Geometry: final body of the model. Coordinates: model frame, mm. Face numbers are marked on the shaded views. A direction names the side the tool comes from. Give positions to 0.01 mm unless a question says otherwise; leave off trailing zeros. Write each loop counter-clockwise with the first axis right and the second up, starting at its lowest first coordinate (ties: lowest second). Pieces come first, ordered by that corner, then holes.
Autodesk Inventor part; units mm, degrees
ref_plane "YZ Plane" through (0, 0, 0) normal (1, 0, 0) x (0, 1, 0)
ref_plane "XZ Plane" through (0, 0, 0) normal (0, 1, 0) x (-1, 0, 0)
ref_plane "XY Plane" through (0, 0, 0) normal (0, 0, 1) x (1, 0, 0)
sketch "Sketch1" plane through (0, 0, 0) normal (0, 0, 1) x (1, 0, 0)
  line L0 (0, 0) -> (0, 40)
  dimension "d0" = 40
sketch "Sketch2" plane through (0, 0, 0) normal (0, 1, 0) x (-1, 0, 0)
  circle A0 centre (0, 0) radius 15
  dimension "d3" = 30
sweep "Sweep1" add profiles "Sketch2" path "Sketch1"
sketch "Sketch4" plane through (0, 0, 0) normal (1, 0, 0) x (0, 1, 0)
  line L0 (0, 17.5) -> (0, -17.5) construction
  line L1 (10, 17.5) -> (10, -17.5)
  line L2 (-10, -17.5) -> (-10, 17.5)
  arc A0 (10, 17.5) -> (-10, 17.5) centre (0, 17.5) ccw
  arc A1 (-10, -17.5) -> (10, -17.5) centre (0, -17.5) ccw
  line L3 (-10, 0) -> (10, 0)
  point P0 (0, 0)
  dimension "d9" = 35
  dimension "d10" = 10
revolve "Revolution1" add sketch "Sketch4" angle 360 about axis through (0, -10, 0) along (0, 1, 0) contours L1 L3 L2 A0
sketch "Sketch5" plane through (0, 0, 0) normal (0, 0, 1) x (1, 0, 0)
  line L0 (-30, 40) -> (30, 40)
  line L1 (30, 40) -> (30, 120)
  line L2 (30, 120) -> (-30, 120)
  line L3 (-30, 120) -> (-30, 40)
  circle A0 centre (0, 90) radius 12.5
  line L4 (0, 0) -> (0, 40) construction
  line L5 (0, 90) -> (0, 40)
  dimension "d12" = 90
  dimension "d13" = 25
  dimension "d14" = 60
  dimension "d15" = 30
extrude "Extrusion1" add sketch "Sketch5" along normal mid plane 80
sketch "Sketch7" plane through (-30, 40, 40) normal (-1, 0, 0) x (0, 0, 1)
  line L0 (-80, 80) -> (0, 80) construction
  line L1 (-65, 80) -> (-15, 80)
  line L2 (-15, 80) -> (-15, 20)
  line L3 (-15, 20) -> (-65, 20)
  line L4 (-65, 20) -> (-65, 80)
  line L5 (-80, 37.5) -> (-80, 62.5) construction
  line L6 (0, 62.5) -> (0, 37.5) construction
  line L7 (-80, 0) -> (-80, 80) construction
  line L8 (-80, 50) -> (0, 50) construction
  line L9 (0, 80) -> (0, 0) construction
  line L10 (-40, 50) -> (-40, 0) construction
  point P0 (-40, -40)
  dimension "d18" = 30
  dimension "d19" = 50
  dimension "d20" = 25
  dimension "d21" = 90
fillet "Fillet1" radius 10 13 edges at (-30, 80, 40) (30, 80, 40) (-30, 80, -40) (30, 80, -40) (-30, 40, 0) (0, 40, -40) (0, 40, 40) (30, 40, 0) (15, 40, 0) (-30, 120, 0) (0, 120, 40) (30, 120, 0) (0, 120, -40)
extrude "Extrusion2" cut sketch "Sketch7" against normal through all
equation "\"d20\" = 0.5 * d19"
properties part number "Elo-Bola Longo"
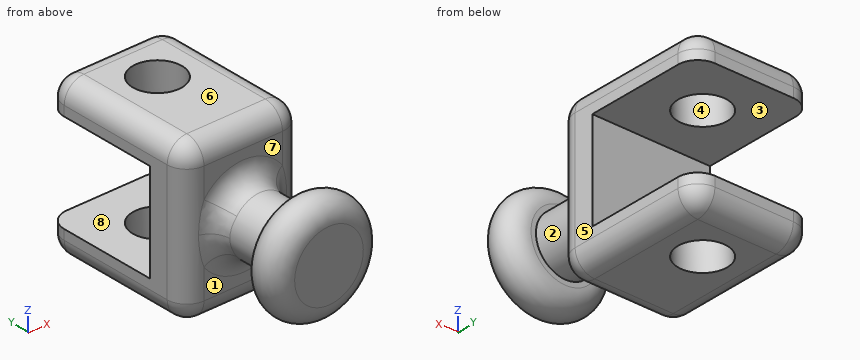
Q1. Ray query, line 1 along Z through (x, y) = (-13, 87); line 2 along Y through (x, z) = (0, 29); line 3 along X through (y, z) = (90, 28). Return the intervals inside material, ascending.
Filled sheet:
line 1: z = -40 to -25, 25 to 40
line 2: y = 40 to 77.5, 102.5 to 120
line 3: x = -30 to -12.5, 12.5 to 30
Q2. Section D-D on y = 25. Output: boundary loops of the cut face in (x, z).
Filled sheet:
outline: circle Ø30 at (0, 0)
Q3. Access query for the marked faces 1, 2, 3, 4 and 5. Directions: +Z, -Z, +X, -X, +Y, -Y. A direction counts if a zero-diameter tool reaches every point of the face in a straight line with its end or side. Return the directions, or none.
Filled sheet:
face 1: -Z
face 2: none
face 3: +X, -X, +Y
face 4: +Z, -Z
face 5: +Z, -Z, +X, +Y, -Y
Q4. Section B-B on x = 0. Count the separate pieces of the cut face and the enclosed holes in it, plus the area to 3 significant figures.
Filled sheet:
separate pieces: 3
enclosed holes: 0
area: 4,520 mm2
Q5. Section C-C on z = 32.5. Output: boundary loops of the cut face in (x, y), plus the area to 3 significant figures.
Filled sheet:
outline: (-29.68, 50) arc R9.68 ccw to (-20, 40.32) - (20, 40.32) arc R9.68 ccw to (29.68, 50) - (29.68, 110) arc R9.68 ccw to (20, 119.68) - (-20, 119.68) arc R9.68 ccw to (-29.68, 110) - close; hole circle Ø25 at (0, 90)
area: 4,140 mm2
Q6. Pin query (flat end, axial travel): P1, Ø2, axis at x = 3, z = -15.5, coming from the +Y side; P2, Ø6, axis at x = 9.5, y = 26, coming from the +Z side; P3, Ø7.5, axis at x = 5, z = -23.5, coming from the -Y side; P4, Ø12, axis at x = 4, z = 22.5, coming from the -Y side. Return the tip coordinate at first contact, or that it passes through.
Filled sheet:
P1: stops at y = 60
P2: stops at z = 13.52
P3: stops at y = -9.61
P4: stops at y = -10
Q7. Pull-direction query (Z, two-part tool) for the marked faces 6, 7 and 8; classes: released by +Z, released by -Z, zero draft, split by the parting line, or undercut.
Filled sheet:
face 6: released by +Z
face 7: zero draft
face 8: undercut
Q8. Section A-A on y = 90. Output: boundary loops of the cut face in (x, z), plus the area to 3 significant figures.
Filled sheet:
outline: (-30, -30) arc R10 ccw to (-20, -40) - (-12.5, -40) - (-12.5, -25) - (-30, -25) - close; (-30, 25) - (-12.5, 25) - (-12.5, 40) - (-20, 40) arc R10 ccw to (-30, 30) - close; (12.5, -40) - (20, -40) arc R10 ccw to (30, -30) - (30, -25) - (12.5, -25) - close; (12.5, 25) - (30, 25) - (30, 30) arc R10 ccw to (20, 40) - (12.5, 40) - close
area: 964 mm2
